The model under review builds one solid part; all positions refer to its coordinate system, in mm. A direction names the side the tool comes from. Round coordinates to 2 decimals unless told otherwise and drop trailing zeros. Write each loop counter-clockwise with the first axis right and the second up, starting at its lowest first coordinate (ties: lowest second). Pieces come first, ordered by that corner, then holes.
Item 1: Add section A-A (z = 0). Give the boundary of the cut face in (x, y), plus the area to 3 significant figures.
Item 2: To check wall thickness, follow L1, parallel to Z at x = 0, y = -23.5; L2, parallel to Z at x = 0, y = 24. State the ranges of each line that lie inside material, in increasing order.
Item 3: Add section D-D (y = -43). Give the boundary of the cut face in (x, z).
Item 4: Clearance check with flat-ended pins moving along their axes: pin 1 Ø1.5 at (y, z) = (34.5, 3) entering from +X; pin 2 Ø2 at (x, z) = (-7.5, 26.5) entering from +Y; pin 3 Ø3 at (x, z) = (-35, -30.5) entering from -Y; pin 4 Ø1 at (y, z) = (32, -31.5) entering from +X (3 decimals). State where each tip first meets the part, or that it passes through.
Item 5: Add section B-B (x = 0). Give the boundary of the cut face in (y, z), plus the area to 3 significant figures.
Item 6: Add section C-C (y = 7). Give the boundary of the cut face in (x, z), plus the area to 3 significant figures.
Item 7: Machinability: for faces 1 (the face through (29.45, -16.874, -9.274)), 2 (the face through (-7.696, 22.308, 34.656)), which of the approach directions +Z, -Z, +X, -X, +Y, -Y give a long, thin tool a straight path to every point of the face, cutting with its end or side? Answer none if there is none.
Item 8: Draft analysis for pull direction X (two halves, no side actions). For faces 3 (the face through (-29.97, -33.72, 1.32)), 4 (the face through (-5.56, -16.87, 25.05)), 5 (the face through (-7, -49, -25)), state which applies: +X half, -X half, draft (parallel to the pull), parting line (faces both ways), or undercut.
Autodesk Inventor part; units mm, degrees
ref_plane "YZ Plane" through (0, 0, 0) normal (1, 0, 0) x (0, 1, 0)
ref_plane "XZ Plane" through (0, 0, 0) normal (0, 1, 0) x (-1, 0, 0)
ref_plane "XY Plane" through (0, 0, 0) normal (0, 0, 1) x (1, 0, 0)
sketch "Sketch1" plane through (0, 0, 0) normal (0, 0, 1) x (1, 0, 0)
  line L0 (0, 0) -> (35.5, 0)
  line L1 (35.5, 0) -> (35.5, 44)
  line L2 (35.5, 44) -> (0, 44)
  line L3 (0, 44) -> (0, 0)
  line L4 (0, 0) -> (0, -18)
  line L5 (0, -18) -> (25, -18)
  line L6 (25, -18) -> (25, -49)
  line L7 (25, -49) -> (0, -49)
  line L8 (0, -49) -> (0, -18)
  line L9 (35.5, 0) -> (25, -18)
  line L10 (0, 0) -> (44, 0)
  line L11 (44, 0) -> (44, 44)
  line L12 (44, 44) -> (0, 44)
  line L13 (0, 44) -> (0, 0)
  line L14 (0, -18) -> (30, -18)
  line L15 (30, -18) -> (30, -49)
  line L16 (30, -49) -> (0, -49)
  line L17 (0, -49) -> (0, -18)
  line L18 (30, -18) -> (44, 0)
  dimension "d13" = 35.5
  dimension "d14" = 44
  dimension "d15" = 18
  dimension "d16" = 25
  dimension "d17" = 31
  dimension "d18" = 44
  dimension "d19" = 30
revolve "Revolution1" add sketch "Sketch1" angle 360 about axis through (0, -49, 0) along (0, 1, 0) contours L10 L18 L14 L9 | L1 L12 L11 L10 | L14 L15 L16 L6
properties part number "PVC_connector" material "PVC-Piping"
Numbers:
1. outline: (-44, 0) - (-30, -18) - (-30, -49) - (-25, -49) - (-25, -18) - (-35.5, 0) - (-35.5, 44) - (-44, 44) - close; (25, -49) - (30, -49) - (30, -18) - (44, 0) - (44, 44) - (35.5, 44) - (35.5, 0) - (25, -18) - close
1. area: 1,300 mm2
2. L1: z = -30 to -25, 25 to 30
2. L2: z = -44 to -35.5, 35.5 to 44
3. outline: circle Ø60 at (0, 0); hole circle Ø50 at (0, 0)
4. pin 1: stops at x = 43.94
4. pin 2: stops at y = -11.93
4. pin 3: passes through
4. pin 4: stops at x = 31.225
5. outline: (-49, -30) - (-18, -30) - (0, -44) - (44, -44) - (44, -35.5) - (0, -35.5) - (-18, -25) - (-49, -25) - close; (-49, 25) - (-18, 25) - (0, 35.5) - (44, 35.5) - (44, 44) - (0, 44) - (-18, 30) - (-49, 30) - close
5. area: 1,300 mm2
6. outline: circle Ø88 at (0, 0); hole circle Ø71 at (0, 0)
6. area: 2,120 mm2
7. face 1: -Y
7. face 2: +Y
8. face 3: parting line
8. face 4: undercut
8. face 5: draft
